Job drawing, mm, ordinate dimensions from the low corner. One solid piece. A direction names the side the tool comes from. Coordinates: 2 decimals unless noted, no trailing zeros. Loops run counter-clockwise (first coordinate to the right, second up) from the corner with the lowest first, then second, coordinate; pieces in that order, holes last. Notation, with made-up numbers: (-28.75, 82.5) - (-8.75, 82.5) arc R8 ccw to (-8.75, 91.5) - close; hole circle Ø1 at (47, 47.25). An arc over 180 degrees is marked (long way). Use a Markdown table: item, result. Add a question column.
1) Tool access for the marked faces 4 and 5: list every direction of +Z, -Z, +X, -X, +Y, -Y with a clear straight run to the whole face (end or side of a thin tool).
2) Band-saw the part on A-A (z = 12.25). Give the cut face in (x, y).
3) Probe probe 1 along X at (y, z) = (9.5, 1.5); probe 2 along Z at (x, y) = (14, 4.5); probe 3 along X at (y, z) = (30.5, 1.75). List the from-to ranges inside material, lowest first. Write a range as [from, to].
4) Band-saw the part on B-B (x = 23.5). Give the cut face in (y, z).
5) Band-saw the part on C-C (z = 4.75). Give the cut face in (x, y).
6) Drop flat-ended pins along their axis: P1, Ø8.5, axis at x = 13, y = 26.5, coming from the -Z side; P2, Ø1.5, axis at x = 3, z = 12.5, coming from the +Y side. Give the stop position or say it passes through.
7) Pull direction Y, two halves, no side cores. Call the marked faces 1, 2 and 3: +Y half, -Y half, draft (parallel to the pull), parting line (faces both ways), or undercut.
8) Band-saw the part on D-D (y = 35.5). Give the cut face in (x, z), plus the area to 3 significant figures.
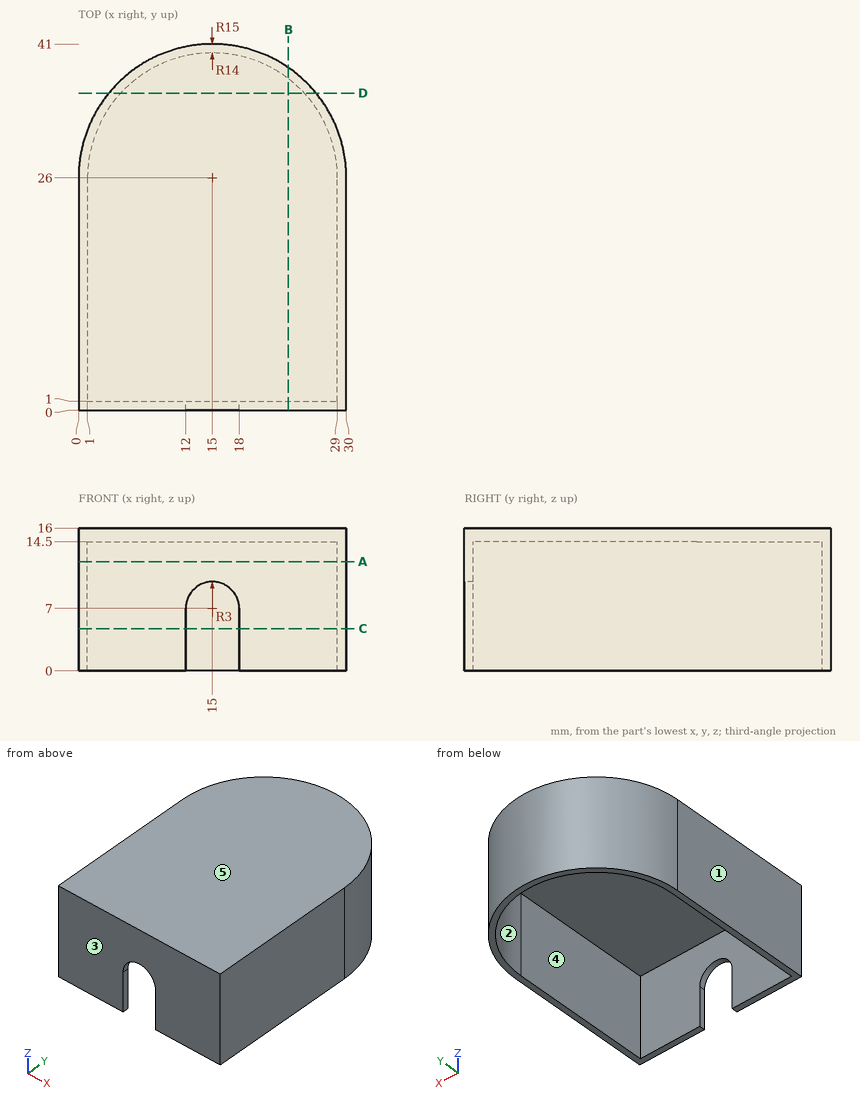
Answer block:
| question | item | result |
|---|---|---|
| 1 | face 4 | -Z |
| 1 | face 5 | +Z, +X, -X, +Y, -Y |
| 2 | outline | (0, 0) - (30, 0) - (30, 26) arc R15 ccw to (0, 26) - close; hole (1, 1) - (29, 1) - (29, 26) arc R14 ccw to (1, 26) - close |
| 3 | probe 1 | [0, 1], [29, 30] |
| 3 | probe 2 | [14.5, 16] |
| 3 | probe 3 | [0.69, 1.74], [28.26, 29.31] |
| 4 | outline | (0, 0) - (1, 0) - (1, 14.5) - (37.12, 14.5) - (37.12, 0) - (38.36, 0) - (38.36, 16) - (0, 16) - close |
| 5 | outline | (0, 0) - (12, 0) - (12, 1) - (1, 1) - (1, 26) arc R14 cw to (29, 26) - (29, 1) - (18, 1) - (18, 0) - (30, 0) - (30, 26) arc R15 ccw to (0, 26) - close |
| 6 | P1 | z = 14.5 |
| 6 | P2 | y = 35.92 |
| 7 | face 1 | draft |
| 7 | face 2 | undercut |
| 7 | face 3 | -Y half |
| 8 | outline | (3.39, 0) - (4.72, 0) - (4.72, 14.5) - (25.28, 14.5) - (25.28, 0) - (26.61, 0) - (26.61, 16) - (3.39, 16) - close |
| 8 | area | 73.2 mm2 |
